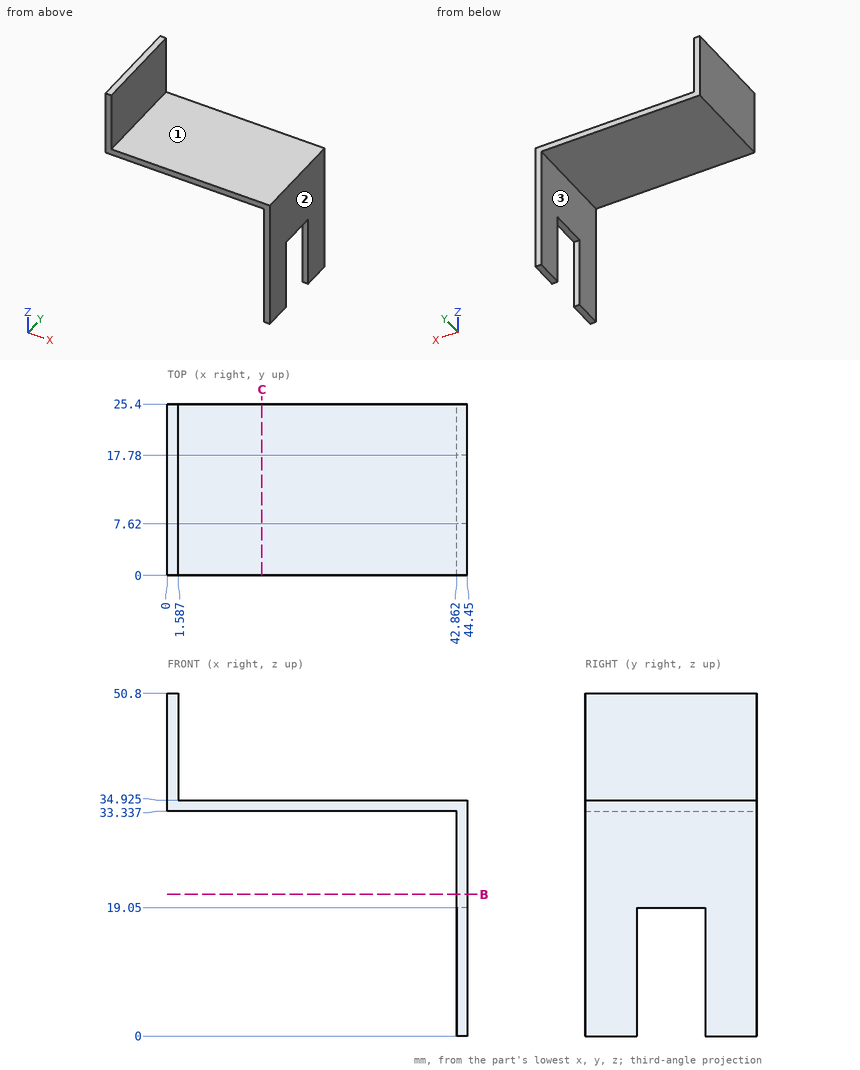
Answer from the drawing. Dimensions are ordinates in mm from the lowest x, y and z of the part. A direction names the side the tool comes from. Give positions to 0.01 mm unless a question says otherwise; leave off trailing zeros. Write each loop counter-clockwise with the first axis right and the second up, starting at its lowest first coordinate (ties: lowest second). Pieces come first, ordered by that corner, then holes.
1) Given P1, Ø12, axis at y = 14.5, z = 27, coming from the -X side; P2, Ø1, axis at x = 35.5, y = 13, coming from the -Z side; P3, Ø1.7, axis at x = 43.5, y = 11.5, coming from the -Z side; P4, Ø6, axis at y = 13.5, z = 13, coming from the -X side, each flat-ended and moving along its own axis, determine where each tip first touches the part or whether it passes through.
2) A tool of negligible diameter and unlimited length cuts with its end or side. For the marked faces 1, 2 and 3, from which of +Z, -Z, +X, -X, +Y, -Y can it reach the whole face along a straight path? Write none if from no direction.
3) Section C-C (x = 14) is taken. Write down the section's boundary in (y, z) (1 decimal).
4) Find the intervals of material crossed by L1, parallel to X at y = 22.5, z = 30.5; L2, parallel to Z at x = 27.5, y = 7.75 (1 decimal); L3, parallel to X at y = 14.25, z = 43.5, in increasing order.
5) Section B-B (z = 21) is taken. Write down the section's boundary in (x, y).
Response:
1. P1: stops at x = 42.86
1. P2: stops at z = 33.34
1. P3: stops at z = 19.05
1. P4: passes through
2. face 1: +Z, +X, +Y, -Y
2. face 2: +Z, -Z, +X, +Y, -Y
2. face 3: -Z, -X, +Y, -Y
3. outline: (0, 33.3) - (25.4, 33.3) - (25.4, 34.9) - (0, 34.9) - close
4. L1: x = 42.86 to 44.45
4. L2: z = 33.3 to 34.9
4. L3: x = 0 to 1.59
5. outline: (42.86, 0) - (44.45, 0) - (44.45, 25.4) - (42.86, 25.4) - close
